Verification items for the finished model (mm, model axes). A direction names the side the tool comes from. Round coordinates to 2 decimals unless told otherwise and drop trailing zeros. Write each loop counter-clockwise with the first axis right and the second up, starting at its lowest first coordinate (ties: lowest second). Pieces come first, ordered by that corner, then holes. Notation, with made-up numbers: (-39.75, 20.25) - (15.25, 20.25) arc R21 ccw to (15.25, 51.25) - close; hole circle Ø11 at (-2.5, 86). An arc over 180 degrees is marked (long way). Write each question's results on one line, items separated by ' | '.
```python
from build123d import *

# Parameters (mm, degrees)
SKETCH2_W                = 85
SKETCH2_H                = 32
BOSS_EXTRUDE1_DEPTH      = 2
EXTRUDE_THIN1_DEPTH      = 2
EXTRUDE_THIN1_DEPTH_BACK = 30
SKETCH2_2_W              = 89
SKETCH2_2_H              = 36
SKETCH2_2_W_2            = 85
SKETCH2_2_H_2            = 32
SKETCH3_W                = 5
SKETCH3_H                = 32
BOSS_EXTRUDE2_DEPTH      = 10
SKETCH4_R                = 2
CUT_EXTRUDE1_DEPTH       = 66.501908369


with BuildPart() as part:
    # Sketch2 → Boss-Extrude1 (new body)
    with BuildSketch(Plane(origin=(0, 0, 0), x_dir=(1, 0, 0), z_dir=(0, 1, 0))):
        Rectangle(SKETCH2_W, SKETCH2_H)
    extrude(amount=BOSS_EXTRUDE1_DEPTH)

    # Sketch2<2> → Extrude-Thin1 (add, two sides: drawn at the far end of the back side and taken through both)
    with BuildSketch(Plane(origin=(0, 0, 0), x_dir=(1, 0, 0), z_dir=(0, 1, 0)).offset(-EXTRUDE_THIN1_DEPTH_BACK)):
        Rectangle(SKETCH2_2_W, SKETCH2_2_H)
        Rectangle(SKETCH2_2_W_2, SKETCH2_2_H_2, mode=Mode.SUBTRACT)
    extrude(amount=EXTRUDE_THIN1_DEPTH + EXTRUDE_THIN1_DEPTH_BACK)

    # Sketch3 → Boss-Extrude2 (add)
    with BuildSketch(Plane(origin=(44.5, 0, 0), x_dir=(0, 0, -1), z_dir=(1, 0, 0))):
        with Locations((0, -14)):
            Rectangle(SKETCH3_W, SKETCH3_H)
    boss_extrude2 = extrude(amount=BOSS_EXTRUDE2_DEPTH)

    # Sketch4 → Cut-Extrude1 (cut, through all)
    with BuildSketch(Plane.XY.offset(2.5)):
        with Locations((49.5, -6)):
            Circle(SKETCH4_R)
        with Locations((49.5, -22)):
            Circle(SKETCH4_R)
    cut_extrude1 = extrude(amount=-CUT_EXTRUDE1_DEPTH, mode=Mode.SUBTRACT)

    # Mirror1: Boss-Extrude2, Cut-Extrude1 across plane
    add(boss_extrude2.mirror(Plane(origin=(0, 0, 0), x_dir=(0, 0, 1), z_dir=(1, 0, 0))))
    add(cut_extrude1.mirror(Plane(origin=(0, 0, 0), x_dir=(0, 0, 1), z_dir=(1, 0, 0))), mode=Mode.SUBTRACT)


solid = part.part
```
(1) Go/stop test with flat-tipped pins: pin 1 Ø12 at (x, z) = (-8, 9) entering from -Y; pin 2 Ø12 at (y, z) = (-2, 9) entering from +X; pin 3 Ø17 at (y, z) = (-9.5, -12.5) entering from -X. Record where each tip stops, or that it passes through.
Answer:
pin 1: y = 0 | pin 2: x = 44.5 | pin 3: x = -44.5
(2) Section check D-D (z = 10.5). Record the cut outline in (x, y), plus the area to 3 significant figures.
Answer:
outline: (-44.5, -30) - (-42.5, -30) - (-42.5, 0) - (42.5, 0) - (42.5, -30) - (44.5, -30) - (44.5, 2) - (-44.5, 2) - close | area: 298 mm2
(3) Set-up check for faces 4 (the flat face through (44.5, -14, -10)), 5 (the flat face through (42.5, -15, 0)), 6 (the flat face through (-44.5, -14, 10)): record each of +Z, -Z, +X, -X, +Y, -Y from which the full face is reachable in a straight line by a thin tool's end or side.
Answer:
face 4: -Z, +X, +Y, -Y | face 5: -Y | face 6: +Z, -X, +Y, -Y
(4) Thickness scan on L1, parallel to Y at x = -49.5, z = 1; L2, parallel to Z at x = 22.5, y = -23.5; L3, parallel to X at y = -10, z = -9. Record the ranges inside material, lowest first.
Answer:
L1: -30 to -24, -20 to -8, -4 to 2 | L2: -18 to -16, 16 to 18 | L3: -44.5 to -42.5, 42.5 to 44.5
(5) Section check B-B (x = -49.5). Record the cut outline in (y, z).
Answer:
outline: (-30, -2.5) - (-24, -2.5) - (-24, 2.5) - (-30, 2.5) - close; (-20, -2.5) - (-8, -2.5) - (-8, 2.5) - (-20, 2.5) - close; (-4, -2.5) - (2, -2.5) - (2, 2.5) - (-4, 2.5) - close
(6) Mould release check, pull along Y, two halves, no side actions. Record for faces 1 (the flat face through (-1, -14, 18)), 2 (the flat face through (-1, 0, 0)), 3 (the cylindrical face through (49.24, -20.017, 0.035)): released by +Y, released by -Y, zero draft, split by the parting line, or undercut.
Answer:
face 1: zero draft | face 2: released by -Y | face 3: undercut
(7) Section check C-C (y = -16.5). Record the cut outline in (x, z).
Answer:
outline: (-54.5, -2.5) - (-44.5, -2.5) - (-44.5, -18) - (44.5, -18) - (44.5, -2.5) - (54.5, -2.5) - (54.5, 2.5) - (44.5, 2.5) - (44.5, 18) - (-44.5, 18) - (-44.5, 2.5) - (-54.5, 2.5) - close; hole (-42.5, -16) - (42.5, -16) - (42.5, 16) - (-42.5, 16) - close
(8) Section check A-A (y = -6). Record the cut outline in (x, z).
Answer:
outline: (-54.5, -2.5) - (-51.5, -2.5) - (-51.5, 2.5) - (-54.5, 2.5) - close; (-47.5, -2.5) - (-44.5, -2.5) - (-44.5, -18) - (44.5, -18) - (44.5, -2.5) - (47.5, -2.5) - (47.5, 2.5) - (44.5, 2.5) - (44.5, 18) - (-44.5, 18) - (-44.5, 2.5) - (-47.5, 2.5) - close; (51.5, -2.5) - (54.5, -2.5) - (54.5, 2.5) - (51.5, 2.5) - close; hole (-42.5, -16) - (42.5, -16) - (42.5, 16) - (-42.5, 16) - close
